Check sheet for the drawn part. Datum: minimum x, y, z corner. Units: mm. Give positions to 0.01 mm unless a question says otherwise; leave off trailing zeros. Loops run counter-clockwise (first coordinate to the right, second up) from the corner with the lowest first, then second, coordinate; pieces in that order, holes last. Notation, with made-up numbers: M 58.5,63.25 L 100.5,63.25 A26 cw 100.5,99.25 Z; hole C 23,69.5 d11. An arc over 180 degrees is marked long. Write each question's results on one line, items separated by ' | '. Start each with the question number.
1. Sectioned sample at A-A on y = 99. Record the cut outline in (x, z), and give its area (3 significant figures).
2. Go/stop test with flat-tipped pins: pin 1 (1.5 mm diameter, centred on y = 104, z = 2, fed in from +X); pin 2 (1.5 mm diameter, centred on x = 1.5, z = 1.5, fed in from +Y). Record where each tip stops, or that it passes through.
3. Material ranges on line 1 along X through (y, z) = (68, 1.7), recorded low to high.
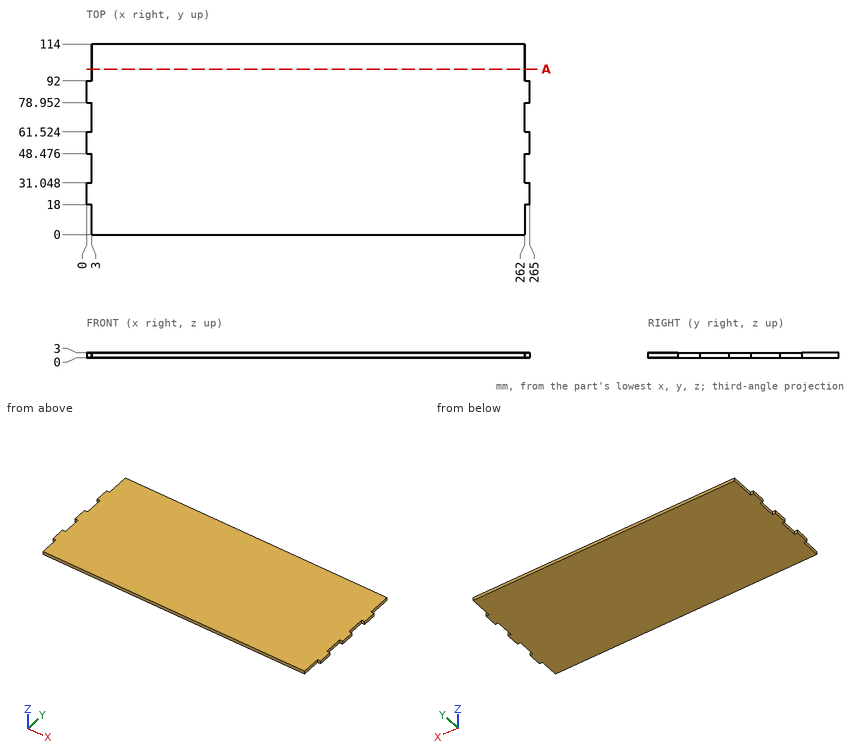
Output values:
1) outline: M 3,0 L 262,0 L 262,3 L 3,3 Z | area: 777 mm2
2) pin 1: x = 262 | pin 2: y = 92
3) line 1: 3 to 262
